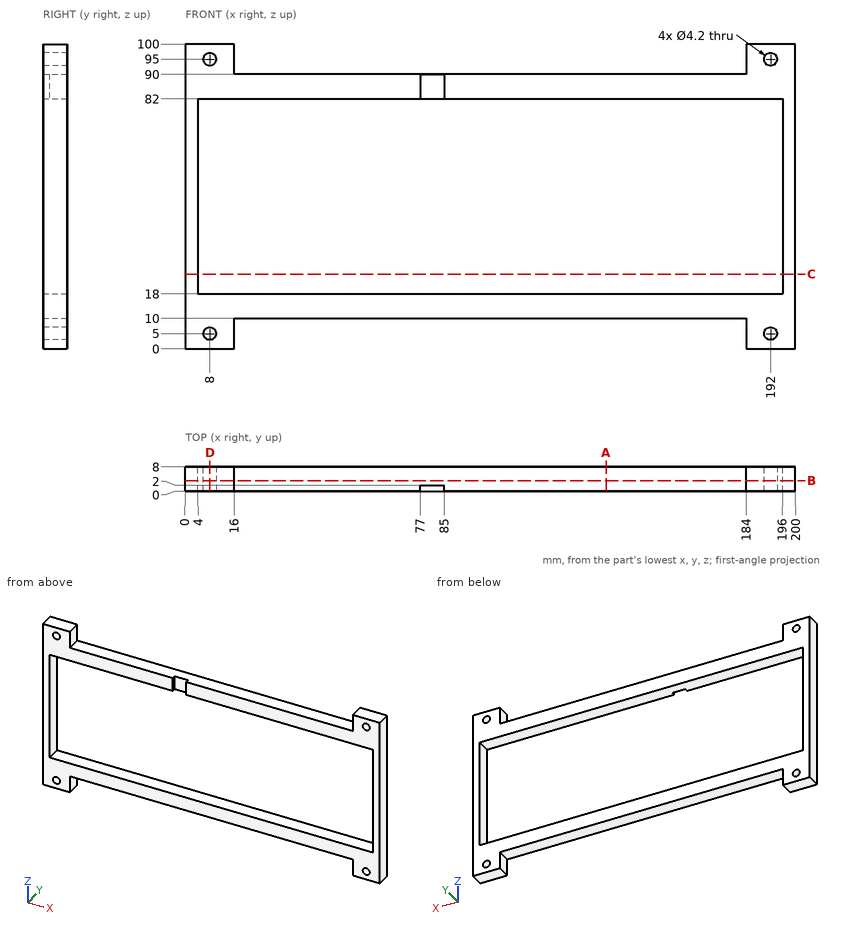
Check sheet for the drawn part. Datum: minimum x, y, z corner. Units: mm. Round coordinates to 2 decimals unless told otherwise and drop trailing zeros. Order: outer loops, then holes, each group sorted by start corner. A loop starts at its lowest first (then second) coordinate and runs counter-clockwise, first axis right, second up. Notation, with made-up numbers: (6, 41.25) -> (40, 41.25) arc R20 cw to (40, 52.25) -> close; hole circle Ø11 at (41.5, -12.5). An arc over 180 degrees is marked (long way). Use CSV: the item, a comma, the result in double quotes.
(1) Cross-section at A-A (x = 138). Record the boundary of the cut face in (y, z), and give its area (3 significant figures).
Worked out:
outline,"(0, 10) -> (8, 10) -> (8, 18) -> (0, 18) -> close; (0, 82) -> (8, 82) -> (8, 90) -> (0, 90) -> close"
area,"128 mm²"
(2) Cross-section at D-D (x = 8). Record the boundary of the cut face in (y, z), and give its area (3 significant figures).
Worked out:
outline,"(0, 0) -> (8, 0) -> (8, 2.9) -> (0, 2.9) -> close; (0, 7.1) -> (8, 7.1) -> (8, 18) -> (0, 18) -> close; (0, 82) -> (8, 82) -> (8, 92.9) -> (0, 92.9) -> close; (0, 97.1) -> (8, 97.1) -> (8, 100) -> (0, 100) -> close"
area,"221 mm²"
(3) Cross-section at C-C (z = 24.5). Record the boundary of the cut face in (x, y), and give its area (3 significant figures).
Worked out:
outline,"(0, 0) -> (4, 0) -> (4, 8) -> (0, 8) -> close; (196, 0) -> (200, 0) -> (200, 8) -> (196, 8) -> close"
area,"64.0 mm²"
(4) Material ranges on line 1 along Z through (x, y) = (192, 5.5); line 2 along Z through (x, y) = (113, 0.5); line 3 along X through (y, z) = (7.75, 75.5), recorded low to high. Write a range as from..to.
Worked out:
line 1,"0..2.9, 7.1..18, 82..92.9, 97.1..100"
line 2,"10..18, 82..90"
line 3,"0..4, 196..200"
(5) Depth check by flat-ended pin: pin 1 (2 mm diameter, centred on x = 54, y = 1, fed in from +Z); pin 2 (6.5 mm diameter, centred on x = 79.5, z = 87, fed in from -Y); pin 3 (2.5 mm diameter, centred on x = 192, z = 95, fed in from -Y); pin 4 (2.5 mm diameter, centred on x = 117, y = 4, fed in from -Z). Enter the tip coordinate at first touch or a pass-through.
Worked out:
pin 1,"z = 90"
pin 2,"y = 0"
pin 3,"through"
pin 4,"z = 10"
(6) Cross-section at B-B (y = 3.5). Record the boundary of the cut face in (x, z), and give its area (3 significant figures).
Worked out:
outline,"(0, 0) -> (16, 0) -> (16, 10) -> (184, 10) -> (184, 0) -> (200, 0) -> (200, 100) -> (184, 100) -> (184, 90) -> (16, 90) -> (16, 100) -> (0, 100) -> close; hole (4, 18) -> (196, 18) -> (196, 82) -> (4, 82) -> close; hole circle Ø4.2 at (8, 5); hole circle Ø4.2 at (8, 95); hole circle Ø4.2 at (192, 5); hole circle Ø4.2 at (192, 95)"
area,"4,300 mm²"
